For this review, take the finished solid that the model builds, in its own axes (mm). A direction names the side the tool comes from. Round coordinates to 2 decimals unless told otherwise and drop trailing zeros. Order: outer loops, then holes, each group sorted by start corner. A loop starts at its lowest first (then second) coordinate and runs counter-clockwise, first axis right, second up. Notation, with made-up numbers: (-22, -26) - (-10, -26) arc R22 cw to (-10, -1) - close; hole circle Ø1 at (-4, -35.75). An arc over 180 degrees is marked (long way). One line per item, written item: value.
```python
from build123d import *

# Parameters (mm, degrees)
PAD_DEPTH    = 3.5
PAD001_DEPTH = 3.5
FILLET_R     = 1
FILLET001_R  = 1


with BuildPart() as part:
    # Sketch → Pad (new body)
    with BuildSketch(Plane.XY):
        with BuildLine():
            Line((-2.5, 0), (2.5, 0))
            Line((2.5, 0), (2.5, -20))
            Line((2.5, -20), (5, -20))
            Line((5, 2.5), (5, -20))
            Line((-5, 2.5), (5, 2.5))
            Line((-5, -20), (-5, 2.5))
            Line((-5, -20), (-2.5, -20))
            Line((-2.5, -20), (-2.5, -19.5))
            ThreePointArc((-2.5, -19.5), (0.5, -16.5), (-2.5, -13.5))
            Line((-2.5, -13.5), (-2.5, -5))
            ThreePointArc((-2.5, -5), (-1, -3.5), (-2.5, -2))
            Line((-2.5, -2), (-2.5, 0))
        make_face()
    extrude(amount=PAD_DEPTH)

    # Sketch001 → Pad001 (join)
    with BuildSketch(Plane.XY):
        with BuildLine():
            Line((-10, 0), (0, 0))
            Line((0, 0), (0, 2.5))
            Line((0, 2.5), (-5.5, 2.5))
            ThreePointArc((-5.5, 2.5), (-7, 4), (-8.5, 2.5))
            Line((-8.5, 2.5), (-9.999981, 2.5))
            ThreePointArc((-11.640701, 2.988407), (-10.855917, 2.62469), (-9.999981, 2.5))
            Line((-11.640701, 2.988407), (-15.61717, 5.586038))
            ThreePointArc((-15.61717, 5.586038), (-16.142156, 5.685413), (-16.584319, 5.38545))
            Line((-17.34717, 4.229013), (-16.584319, 5.38545))
            ThreePointArc((-17.34717, 4.229013), (-17.407235, 3.915539), (-17.227457, 3.651808))
            Line((-13.007951, 0.895412), (-17.227457, 3.651808))
            ThreePointArc((-13.007951, 0.895412), (-11.569198, 0.228604), (-10, 0))
        make_face()
    extrude(amount=PAD001_DEPTH)

    # Fillet
    fillet_edges = [part.edges().sort_by_distance(p)[0] for p in [
        (-5, 0, 1.75),
    ]]
    fillet(fillet_edges, radius=FILLET_R)

    # Fillet001
    fillet001_edges = [part.edges().sort_by_distance(p)[0] for p in [
        (5, 2.5, 1.75),
        (5, -20, 1.75),
        (2.5, -20, 1.75),
        (-5, -20, 1.75),
    ]]
    fillet(fillet001_edges, radius=FILLET001_R)


solid = part.part
```
Item 1: For P1, Ø1.8, axis at x = 0.5, z = 2, coming from the -Y side; P2, Ø1, axis at y = -12, z = 1.5, coming from the -X side; P3, Ø1.6, axis at x = -9.5, z = 2.5, coming from the +Y side, all flat-tipped, find the tip position at first contact; note any pin that passes through.
Returned:
P1: y = -18.64
P2: x = -5
P3: y = 2.52
Item 2: Take a section at C-C (y = -8). Write out the cut boundary in (x, z).
Returned:
outline: (-5, 0) - (-2.5, 0) - (-2.5, 3.5) - (-5, 3.5) - close; (2.5, 0) - (5, 0) - (5, 3.5) - (2.5, 3.5) - close
Item 3: Take a section at B-B (z = 1.8). Write out the cut boundary in (x, y), plus the area to 3 significant figures.
Returned:
outline: (-17.35, 4.23) arc R0.42 ccw to (-17.23, 3.65) - (-13.01, 0.9) arc R5.5 ccw to (-10, 0) - (-6, 0) arc R1 cw to (-5, -1) - (-5, -19) arc R1 ccw to (-4, -20) - (-2.5, -20) - (-2.5, -19.5) arc R3 ccw to (-2.5, -13.5) - (-2.5, -5) arc R1.5 ccw to (-2.5, -2) - (-2.5, 0) - (2.5, 0) - (2.5, -19) arc R1 ccw to (3.5, -20) - (4, -20) arc R1 ccw to (5, -19) - (5, 1.5) arc R1 ccw to (4, 2.5) - (-5.5, 2.5) arc R1.5 ccw to (-8.5, 2.5) - (-10, 2.5) arc R3 cw to (-11.64, 2.99) - (-15.62, 5.59) arc R0.7 ccw to (-16.58, 5.39) - close
area: 178 mm^2
Item 4: Wall thickness on line 1 (X direction, y = -8, z = 0.25); line 2 (X direction, y = -16, z = 1.35); line 3 (Y direction, x = 1.5, z = 1): over which ranges is each line inside the solid? List them lowest first.
Returned:
line 1: -5 to -2.5, 2.5 to 5
line 2: -5 to 0.46, 2.5 to 5
line 3: 0 to 2.5
Item 5: Machinability: for faces 5 (the flat face through (-8, 0, 2)), 6 (the cylindrical face through (2.785, -19.699, 1.774)), 7 (the flat face through (-9, 2.5, 2)), which of the approach directions +Z, -Z, +X, -X, +Y, -Y give a long, thin tool a straight path to every point of the face, cutting with its end or side? Answer none if there is none.
Returned:
face 5: +Z, -Z, -X, -Y
face 6: +Z, -Z, -Y
face 7: +Z, -Z, +Y
Item 6: Take a section at A-A (y = -16.5). Write out the cut boundary in (x, z).
Returned:
outline: (-5, 0) - (0.5, 0) - (0.5, 3.5) - (-5, 3.5) - close; (2.5, 0) - (5, 0) - (5, 3.5) - (2.5, 3.5) - close
Item 7: Take a section at D-D (x = -10.5). Write out the cut boundary in (y, z), plus the area to 3 significant figures.
Returned:
outline: (0.02, 0) - (2.54, 0) - (2.54, 3.5) - (0.02, 3.5) - close
area: 8.82 mm^2
Item 8: The part is to be moulded in two halves that separate along Y. For faces 1 (the cylindrical face through (-16.135, 5.687, 1.726)), 2 (the cylindrical face through (4.699, -19.715, 1.774)), 3 (the flat face through (0, 0, 2)), 4 (the flat face through (-4, -6, 3.5)), say which applies: +Y half, -Y half, draft (parallel to the pull), parting line (faces both ways), or undercut.
Returned:
face 1: +Y half
face 2: -Y half
face 3: undercut
face 4: draft
